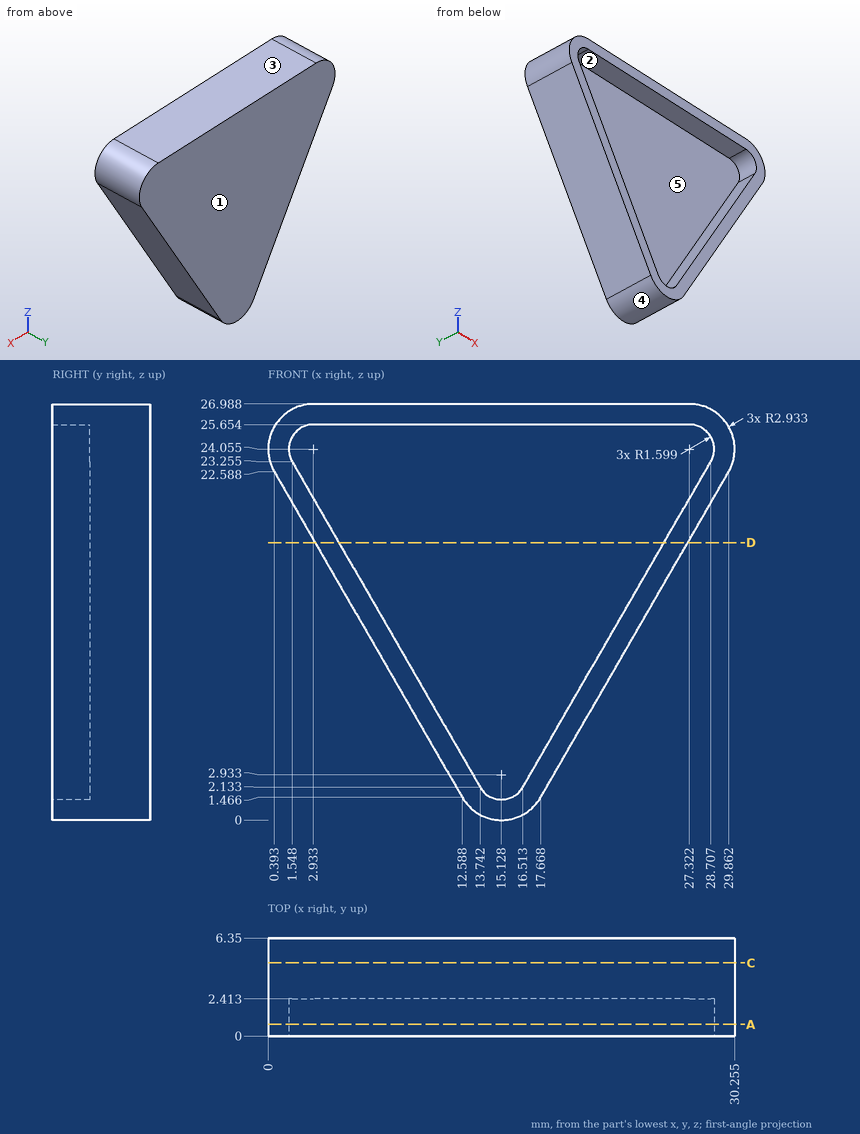
Answer from the drawing. Dimensions are ordinates in mm from the lowest x, y and z of the part. A direction names the side the tool comes from. Give positions to 0.01 mm unless a question says otherwise; leave off trailing zeros. Write each loop counter-clockwise with the first axis right and the second up, starting at its lowest first coordinate (ties: lowest second). Pieces come first, ordered by that corner, then holes.
1) Section C-C (y = 4.75) is taken. Write down the section's boundary in (x, z) (1 decimal).
2) Given P1, Ø6, axis at x = 13.5, z = 21.5, coming from the -Y side; P2, Ø2, axis at y = 5, z = 6, coming from the -X side; P3, Ø3, axis at y = 3.5, z = 6.5, coming from the -X side (1 decimal); P4, Ø12, axis at x = 15, z = 3.5, coming from the -Y side, each flat-ended and moving along its own axis, determine where each tip first touches the part or whether it passes through.
3) For a pull along Z with two mould halves and no side action, classify the marked faces 3, 4 and 5 as pulls with the +Z half, pulls with the -Z half, needs draft (parallel to the pull), parting line crosses it, or undercut.
4) Section A-A (y = 0.75) is taken. Write down the section's boundary in (x, z) (1 decimal).
5) Find the intervals of material crossed by L1, parallel to Y at x = 23, z = 25.5; L2, parallel to Z at x = 15.5, y = 0.75 (1 decimal); L3, parallel to X at y = 0.5, z = 8 (1 decimal), in increasing order.
6) A tool of negligible diameter and unlimited length cuts with its end or side. For the marked faces 1 and 2, from which of +Z, -Z, +X, -X, +Y, -Y can it reach the whole face along a straight path? Write none if from no direction.
7) Section D-D (z = 18) is taken. Write down the section's boundary in (x, y), and give its area (3 significant figures).
Response:
1. outline: (0.4, 22.6) - (12.6, 1.5) arc R2.9 ccw to (17.7, 1.5) - (29.9, 22.6) arc R2.9 ccw to (27.3, 27) - (2.9, 27) arc R2.9 ccw to start
2. P1: stops at y = 2.41
2. P2: stops at x = 9.39
2. P3: stops at x = 8.8
2. P4: stops at y = 0
3. face 3: pulls with the +Z half
3. face 4: pulls with the -Z half
3. face 5: undercut
4. outline: (0.4, 22.6) - (12.6, 1.5) arc R2.9 ccw to (17.7, 1.5) - (29.9, 22.6) arc R2.9 ccw to (27.3, 27) - (2.9, 27) arc R2.9 ccw to start; hole (1.5, 23.3) - (13.7, 2.1) arc R1.6 ccw to (16.5, 2.1) - (28.7, 23.3) arc R1.6 ccw to (27.3, 25.7) - (2.9, 25.7) arc R1.6 ccw to start
5. L1: y = 2.41 to 6.35
5. L2: z = 0 to 1.4, 25.7 to 27
5. L3: x = 8.8 to 10.4, 19.9 to 21.4
6. face 1: +Z, -Z, +X, -X, +Y
6. face 2: -Y
7. outline: (3.04, 0) - (4.58, 0) - (4.58, 2.41) - (25.67, 2.41) - (25.67, 0) - (27.21, 0) - (27.21, 6.35) - (3.04, 6.35) - close
7. area: 103 mm2
